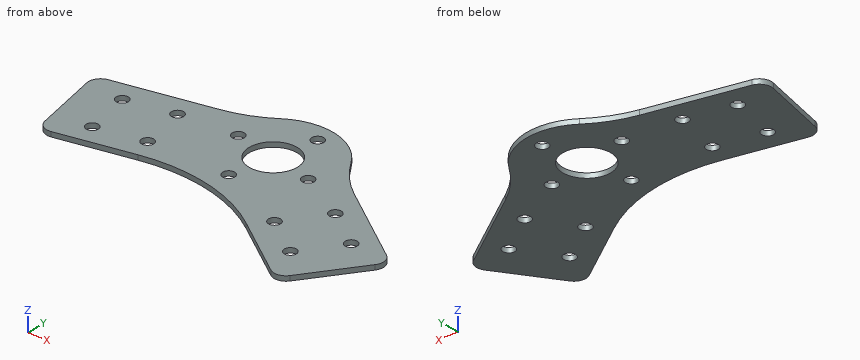
```python
from build123d import *

# Parameters (mm, degrees)
SKETCH1_R           = 2.5
SKETCH1_R_2         = 10
BOSS_EXTRUDE1_DEPTH = 2
FILLET1_R           = 50
FILLET2_R           = 70
FILLET3_R           = 5


with BuildPart() as part:
    # Sketch1 → Boss-Extrude1 (new body)
    with BuildSketch(Plane.XY):
        with BuildLine():
            Line((-77.311392181, 2.991427603), (-69.410747929, -34.178181225))
            Line((-69.410747929, -34.178181225), (-4.13058082, -20.302453359))
            Line((-4.13058082, -20.302453359), (50.538451031, -58.582121568))
            Line((50.538451031, -58.582121568), (72.334355612, -27.454343885))
            Line((72.334355612, -27.454343885), (24.207597625, 6.244374848))
            ThreePointArc((24.207597625, 6.244374848), (4.98419836, 24.498117616), (-19.843339473, 15.206639292))
            Line((-19.843339473, 15.206639292), (-77.311392181, 2.991427603))
        make_face()
        with Locations((-60.767972952, -2.693225442)):
            Circle(SKETCH1_R, mode=Mode.SUBTRACT)
        with Locations((-56.609739136, -22.256177456)):
            Circle(SKETCH1_R, mode=Mode.SUBTRACT)
        with Locations((-37.046787121, -18.09794364)):
            Circle(SKETCH1_R, mode=Mode.SUBTRACT)
        with Locations((-41.205020938, 1.465008375)):
            Circle(SKETCH1_R, mode=Mode.SUBTRACT)
        with Locations((38.501846135, -14.751537011)):
            Circle(SKETCH1_R, mode=Mode.SUBTRACT)
        with Locations((27.030317408, -31.134577897)):
            Circle(SKETCH1_R, mode=Mode.SUBTRACT)
        with Locations((43.413358294, -42.606106624)):
            Circle(SKETCH1_R, mode=Mode.SUBTRACT)
        with Locations((54.884887021, -26.223065738)):
            Circle(SKETCH1_R, mode=Mode.SUBTRACT)
        Circle(SKETCH1_R_2, mode=Mode.SUBTRACT)
        with Locations((3.58862282, 17.638644683)):
            Circle(SKETCH1_R, mode=Mode.SUBTRACT)
        with Locations((17.638644683, -3.58862282)):
            Circle(SKETCH1_R, mode=Mode.SUBTRACT)
        with Locations((-3.58862282, -17.638644683)):
            Circle(SKETCH1_R, mode=Mode.SUBTRACT)
        with Locations((-17.638644683, 3.58862282)):
            Circle(SKETCH1_R, mode=Mode.SUBTRACT)
    extrude(amount=BOSS_EXTRUDE1_DEPTH)

    # Fillet1
    fillet1_edges = [part.edges().sort_by_distance(p)[0] for p in [
        (-19.843339473, 15.206639292, 1),
        (24.207597625, 6.244374848, 1),
    ]]
    fillet(fillet1_edges, radius=FILLET1_R)

    # Fillet2
    fillet2_edges = [part.edges().sort_by_distance(p)[0] for p in [
        (-4.13058082, -20.302453359, 1),
    ]]
    fillet(fillet2_edges, radius=FILLET2_R)

    # Fillet3
    fillet3_edges = [part.edges().sort_by_distance(p)[0] for p in [
        (72.334355612, -27.454343885, 1),
        (50.538451031, -58.582121568, 1),
        (-69.410747929, -34.178181225, 1),
        (-77.311392181, 2.991427603, 1),
    ]]
    fillet(fillet3_edges, radius=FILLET3_R)


solid = part.part
```
The model under review builds one solid part; all positions refer to its coordinate system, in mm. Round coordinates to 2 decimals unless told otherwise and drop trailing zeros. Order: outer loops, then holes, each group sorted by start corner. A loop starts at its lowest first (then second) coordinate and runs counter-clockwise, first axis right, second up. Notation, with made-up numbers: (-38, 4.25) - (-15, 4.25) arc R18 cw to (-15, 24.25) - close; hole circle Ø2 at (66, 9.25). An arc over 180 degrees is marked (long way). Answer in a Markdown table with one row per item.
(1) Take a section at A-A on x = -56. Write out the cut boundary in (y, z).
Result set:
| item | result |
|---|---|
| outline | (-31.33, 0) - (-24.68, 0) - (-24.68, 2) - (-31.33, 2) - close; (-19.83, 0) - (7.52, 0) - (7.52, 2) - (-19.83, 2) - close |
(2) Take a section at D-D on x = -23.5. Write out the cut boundary in (y, z).
Result set:
| item | result |
|---|---|
| outline | (-25.22, 0) - (15.38, 0) - (15.38, 2) - (-25.22, 2) - close |
(3) Clearance check with a flat-ended pin moving along its axis: P1, Ø1, axis at x = -60, z = 1.5, coming from the +Y side. State where the tip first meets the part, or that it passes through.
Result set:
| item | result |
|---|---|
| P1 | stops at y = 6.78 |
(4) For line 1 (X direction, y = -24, z = 0.2); line 2 (X direction, y = -9, z = 1.05); line 3 (X direction, y = -6.5, z = 1.35), list the stretches that pass through material, from the lowest coordinate up. Write a range as from..to.
Result set:
| item | result |
|---|---|
| line 1 | x = -71.57..-58.4, -54.82..53.74, 56.03..67.4 |
| line 2 | x = -74.76..-4.36, 4.36..45.98 |
| line 3 | x = -75.29..-7.6, 7.6..42.41 |
(5) Take a section at B-B on z = 0.3. Count the separate pieces of the cut face and the enclosed holes in it, plus the area to 3 significant figures.
Result set:
| item | result |
|---|---|
| separate pieces | 1 |
| enclosed holes | 13 |
| area | 5,510 mm2 |
(6) Take a section at C-C on y = -46.5. Write out the cut boundary in (x, z), plus the area to 3 significant figures.
Result set:
| item | result |
|---|---|
| outline | (33.28, 0) - (59, 0) - (59, 2) - (33.28, 2) - close |
| area | 51.4 mm2 |
